Geometry check sheet. Reference: the model listing, model coordinates, mm. Face numbers are marked on the shaded views. A direction names the side the tool comes from. Coordinates: 2 decimals unless noted, no trailing zeros. Write each loop counter-clockwise with the first axis right and the second up, starting at its lowest first coordinate (ties: lowest second). Pieces come first, ordered by that corner, then holes. Notation, with made-up numbers: (3, 76) -> (30, 76) arc R23 ccw to (30, 88) -> close; hole circle Ø8 at (24, 39.25). An arc over 180 degrees is marked (long way). Put each result on its own line as item: value. Start each with the question number.
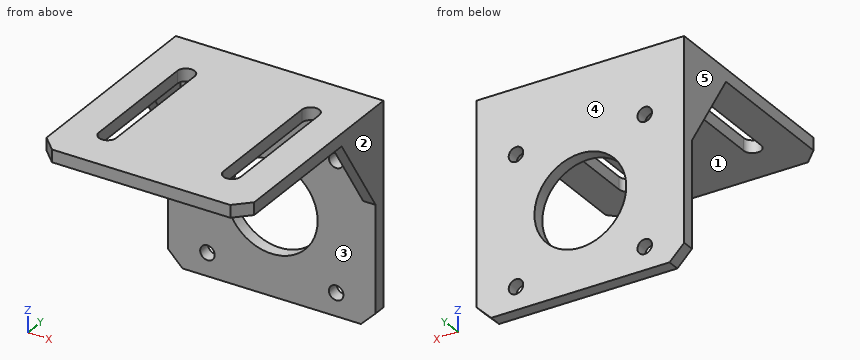
from build123d import *

# Parameters (mm, degrees)
SKETCH_1_R      = 11.05
SKETCH_1_R_2    = 1.75
EXTRUDE_1_DEPTH = 3
EXTRUDE_2_DEPTH = 3
EXTRUDE_3_DEPTH = 3
EXTRUDE_4_DEPTH = 3


with BuildPart() as part:
    # 草图1 → 凸台-拉伸1 (new body)
    with BuildSketch(Plane(origin=(0, 0, 0), x_dir=(1, 0, 0), z_dir=(0, 1, 0))):
        Polygon((0, 0), (0, 45.464466094), (3.535533906, 49), (46.464466094, 49), (50, 45.464466094), (50, 0), align=None)
        with Locations(Location((25, 28, 0), (0, 0, 270))):
            Circle(SKETCH_1_R, mode=Mode.SUBTRACT)
        with Locations(Location((9.5, 12.5, 0), (0, 0, 270))):
            Circle(SKETCH_1_R_2, mode=Mode.SUBTRACT)
        with Locations(Location((9.5, 43.5, 0), (0, 0, 270))):
            Circle(SKETCH_1_R_2, mode=Mode.SUBTRACT)
        with Locations(Location((40.5, 43.5, 0), (0, 0, 270))):
            Circle(SKETCH_1_R_2, mode=Mode.SUBTRACT)
        with Locations(Location((40.5, 12.5, 0), (0, 0, 270))):
            Circle(SKETCH_1_R_2, mode=Mode.SUBTRACT)
    extrude(amount=EXTRUDE_1_DEPTH)

    # 草图2 → 凸台-拉伸2 (add)
    with BuildSketch(Plane.XY):
        Polygon((0, 3), (0, -46.464466094), (3.535533906, -50), (46.464466094, -50), (50, -46.464466094), (50, 3), align=None)
        with BuildLine():
            Line((12.1, -9), (12.1, -39))
            ThreePointArc((12.1, -39), (10, -41.1), (7.9, -39))
            Line((7.9, -39), (7.9, -9))
            ThreePointArc((7.9, -9), (10, -6.9), (12.1, -9))
        make_face(mode=Mode.SUBTRACT)
        with BuildLine():
            Line((37.9, -9), (37.9, -39))
            ThreePointArc((37.9, -39), (40, -41.1), (42.1, -39))
            Line((42.1, -39), (42.1, -9))
            ThreePointArc((42.1, -9), (40, -6.9), (37.9, -9))
        make_face(mode=Mode.SUBTRACT)
    extrude(amount=EXTRUDE_2_DEPTH)

    # 草图3 → 凸台-拉伸3 (add)
    with BuildSketch(Plane(origin=(50, 0, 0), x_dir=(0, 0, -1), z_dir=(1, 0, 0))):
        Polygon((0, 0), (0, -13), (20, 0), align=None)
    extrude(amount=-EXTRUDE_3_DEPTH)

    # 草图4 → 凸台-拉伸4 (add)
    with BuildSketch(Plane.ZY):
        Polygon((-20, 0), (0, 0), (0, -13), align=None)
    extrude(amount=-EXTRUDE_4_DEPTH)


solid = part.part
Item 1: Section check C-C, the plane x = 25. Enter the section's corners in (y, z), and give its area (3 significant figures).
Item 2: Access from +Z, -Z, +X, -X, +Y, -Y to the whole of each face (thin tool, end or side, straight path). Record for the marked faces 1 and 2.
Item 3: Section check A-A, the plane y = -23.5. Enter the section's corners in (x, z), and give its area (3 significant figures).
Item 4: Go/stop test with flat-tipped pins: P1, Ø10.5, axis at y = -6.5, z = -13.5, coming from the +X side; P2, Ø1, axis at x = 20.5, y = -26, coming from the -Z side; P3, Ø12, axis at x = 6.5, z = -36, coming from the -Y side. Record where each tip stops, or that it passes through.
Item 5: Section check B-B, the plane z = -43.5. Enter the section's corners in (x, y).
Item 6: Section check D-D, the plane z = -28. Enter the section's corners in (x, y), and give its area (3 significant figures).
Item 7: Mould release check, pull along X, two halves, no side actions. Record for the marked faces 3, 4 and 5: released by +X, released by -X, zero draft, split by the parting line, or undercut.
Item 8: Scan lines: line 1 along X through (y, z) = (-1.5, -4); line 2 along X through (y, z) = (1, -43); line 3 along Z through (x, y) = (40, 1). Record each from-to range of solid material in increasing order. Write a range as [from, to].
From the geometry:
1. outline: (-50, 0) -> (0, 0) -> (0, -16.95) -> (3, -16.95) -> (3, 3) -> (-50, 3) -> close; (0, -49) -> (3, -49) -> (3, -39.05) -> (0, -39.05) -> close
1. area: 240 mm²
2. face 1: -Z, -Y
2. face 2: +Z, -Z, +X, +Y, -Y
3. outline: (0, 0) -> (7.9, 0) -> (7.9, 3) -> (0, 3) -> close; (12.1, 0) -> (37.9, 0) -> (37.9, 3) -> (12.1, 3) -> close; (42.1, 0) -> (50, 0) -> (50, 3) -> (42.1, 3) -> close
3. area: 125 mm²
4. P1: x = 50
4. P2: z = 0
4. P3: y = 0
5. outline: (0, 0) -> (7.75, 0) -> (7.75, 3) -> (0, 3) -> close; (11.25, 0) -> (38.75, 0) -> (38.75, 3) -> (11.25, 3) -> close; (42.25, 0) -> (50, 0) -> (50, 3) -> (42.25, 3) -> close
6. outline: (0, 0) -> (13.95, 0) -> (13.95, 3) -> (0, 3) -> close; (36.05, 0) -> (50, 0) -> (50, 3) -> (36.05, 3) -> close
6. area: 83.7 mm²
7. face 3: undercut
7. face 4: zero draft
7. face 5: released by -X
8. line 1: [0, 3], [47, 50]
8. line 2: [0, 7.82], [11.18, 38.82], [42.18, 50]
8. line 3: [-49, -45.18], [-41.82, -14.18], [-10.82, 3]
